```python
from build123d import *

# Parameters (mm, degrees)
F3_DEPTH      = 12.7
F4_R          = 10.16
F5_DEPTH      = 138.60962
F5_DEPTH_BACK = 3.74144


with BuildPart() as f1:
    # F0 (on Front) → F1 (revolve)
    with BuildSketch(Plane.XZ):
        with BuildLine():
            Line((-78.6915116169, 11.7242524082), (-86.5560208407, 11.7242524082))
            Line((-86.5560208407, 11.7242524082), (-86.5560208407, 10.1367524082))
            Line((-86.5560208407, 10.1367524082), (-88.1435208407, 10.1367524082))
            Line((-88.1435208407, 10.1367524082), (-88.1435208407, 11.7242524082))
            Line((-88.1435208407, 11.7242524082), (-90.648425594, 11.7242524082))
            Line((-90.648425594, 11.7242524082), (-90.648425594, 10.1367524082))
            Line((-90.648425594, 10.1367524082), (-92.235925594, 10.1367524082))
            Line((-92.235925594, 10.1367524082), (-92.235925594, 11.7242524082))
            ThreePointArc((-92.235925594, 11.7242524082), (-101.2161817151, 8.0045085293), (-104.935925594, -0.9757475918))
            Line((-104.935925594, -0.9757475918), (47.464074406, -0.9757475918))
            Line((47.464074406, -0.9757475918), (61.2039872572, -0.9757475918))
            Line((61.2039872572, -0.9757475918), (61.2039872572, 5.3742524082))
            Line((61.2039872572, 5.3742524082), (47.464074406, 11.7242524082))
            Line((47.464074406, 11.7242524082), (-66.3975579772, 11.7242524082))
            Line((-66.3975579772, 11.7242524082), (-66.3975579772, 10.1367524082))
            Line((-66.3975579772, 10.1367524082), (-67.9850579772, 10.1367524082))
            Line((-67.9850579772, 10.1367524082), (-67.9850579772, 11.7242524082))
            Line((-67.9850579772, 11.7242524082), (-75.5165116169, 11.7242524082))
            Line((-75.5165116169, 11.7242524082), (-75.5165116169, 10.1367524082))
            Line((-75.5165116169, 10.1367524082), (-78.6915116169, 10.1367524082))
            Line((-78.6915116169, 10.1367524082), (-78.6915116169, 11.7242524082))
        make_face()
    revolve(axis=Axis((-28.735925594, 0, -0.9757475918), (-1, 0, 0)))

    # F2 (on Front) → F3 (cut, symmetric)
    with BuildSketch(Plane.XZ):
        with BuildLine():
            ThreePointArc((-56.52696557, 8.2861608072), (-51.8724141542, 2.2753715234), (-44.6186481582, 0))
            Line((-44.6186481582, 0), (25.2313518418, 0))
            ThreePointArc((25.2313518418, 0), (32.6508184362, 2.392647505), (37.2746679855, 8.6690526842))
            ThreePointArc((37.2746679855, 8.6690526842), (39.0418683994, 10.5448245437), (41.3332582144, 11.7242524082))
            Line((41.3332582144, 11.7242524082), (-60.2667417856, 11.7242524082))
            ThreePointArc((-60.2667417856, 11.7242524082), (-58.1019120471, 10.3260286868), (-56.52696557, 8.2861608072))
        make_face()
    extrude(amount=F3_DEPTH, both=True, mode=Mode.SUBTRACT)

    # F4 (on face) → F5 (cut, two sides)
    with BuildSketch(Plane(origin=(-90.648425594, 0, 0), x_dir=(0, -1, 0), z_dir=(-1, 0, 0))) as f5_sk:
        with Locations((0, -0.9757475918)):
            Circle(F4_R)
    extrude(amount=-F5_DEPTH, mode=Mode.SUBTRACT)
    extrude(f5_sk.sketch, amount=F5_DEPTH_BACK, mode=Mode.SUBTRACT)


solid = f1.part
```
Could you check a few things on this model? Use its own coordinates, in mm. A direction names the side the tool comes from. Round coordinates to 2 decimals unless told otherwise and drop trailing zeros. Write each loop counter-clockwise with the first axis right and the second up, starting at its lowest first coordinate (ties: lowest second). Pieces come first, ordered by that corner, then holes. Notation, with made-up numbers: M 20.5,31.5 L 40.5,31.5 A14 cw 40.5,45.5 Z; hole C 86.5,49.25 d1. An arc over 180 degrees is marked long. Answer in a Markdown table with one row per item. Add a question column.
Q1. Imagine slicing it at A-A (x = 16). Please give me the cut outline in (y, z), then the cut area to 3 significant figures.
Q2. Will these pins go through, and if not, where does the flat tip stop? pin 1 Ø1.5 at (x, y) = (38.5, -1) entering from -Z; pin 2 Ø1.3 at (x, y) = (-16, 11) entering from +Z; pin 3 Ø12.5 at (y, z) = (-4.5, 4.5) entering from -X.
Q3. If I drill on line 1 (Y direction, x = -11.5, z = -0.75); line 2 (Z direction, x = -92.95, y = 0); line 3 (Y direction, x = 34.5, z = -10.25), over which ranges is the centre line in solid material (lowest first)? Write a range as from..to.
Q4. On a 3-axis mill with a long thin cutter (end or side, diameter ignored), from which of +Z, -Z, +X, -X, +Y, -Y can I reach the whole of each face in a straight line? I mean faces 5 (the cylindrical face through (-51.961, 10.246, 2.337)), 6 (the cylindrical face through (-89.414, -12.398, -3.729)), 7 (the flat face through (-92.236, -11.23, -1.86)). Say none if no direction works.
Q5. If we mould it in two halves opening along Y, with no side actions, what happens to faces 1 (the flat face through (-86.556, -11.23, -0.09)), 2 (the flat face through (-94.39, 0, -1)), 3 (the cylindrical face through (-10.264, 0.558, -13.663)), 4 (the flat face through (47.961, 0, -1))? For each: +Y half, -Y half, draft (parallel to the pull), parting line (faces both ways), or undercut.
Values:
| question | item | result |
|---|---|---|
| 1 | outline | M -12.66,0 A12.7 ccw long 12.66,0 L 10.11,0 A10.16 cw long -10.11,0 Z |
| 1 | area | 96.2 mm^2 |
| 2 | pin 1 | z = -13.67 |
| 2 | pin 2 | z = 0 |
| 2 | pin 3 | x = -104.91 |
| 3 | line 1 | -12.7..-10.16, 10.16..12.7 |
| 3 | line 2 | -13.66..-11.14, 9.18..11.7 |
| 3 | line 3 | -8.68..-4.15, 4.15..8.68 |
| 4 | face 5 | +Z, +Y, -Y |
| 4 | face 6 | +X, -X |
| 4 | face 7 | none |
| 5 | face 1 | draft |
| 5 | face 2 | undercut |
| 5 | face 3 | parting line |
| 5 | face 4 | undercut |
